Could you check a few things on this model? Use its own coordinates, in mm. Face numbers are marked on the shaded views. A direction names the side the tool comes from. Round coordinates to 2 decimals unless told otherwise and drop trailing zeros. Write each loop counter-clockwise with the first axis right and the second up, starting at its lowest first coordinate (ties: lowest second). Pieces come first, ordered by that corner, then holes. Notation, with made-up numbers: (-21.75, -19.75) - (28.25, -19.75) arc R5 ccw to (28.25, -15.75) - close; hole circle Ø5 at (16, 16). An arc over 180 degrees is marked (long way). Put each result on its own line as item: value.
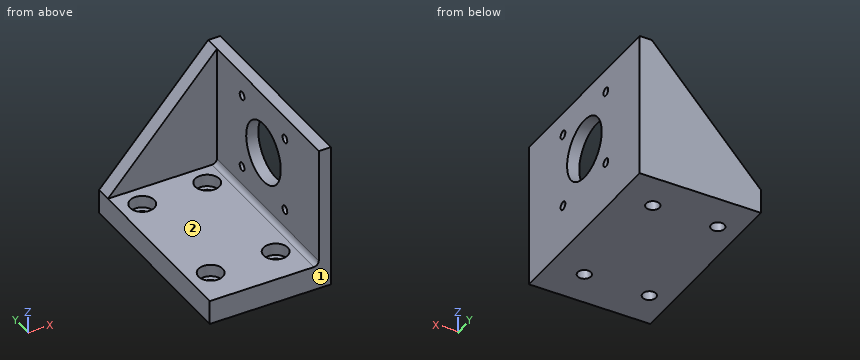
from build123d import *

# Parameters (mm, degrees)
SKETCH1_W                      = 50
SKETCH1_H                      = 80
BOSS_EXTRUDE1_DEPTH            = 10
SKETCH2_W                      = 5
SKETCH2_H                      = 80
BOSS_EXTRUDE2_DEPTH            = 50
SKETCH3_R                      = 12.5
CUT_EXTRUDE1_DEPTH             = 88.749643874
M3_CLEARANCE_HOLE1_D           = 3.4
CBORE_FOR_M5_SHCS1_D           = 5.5
CBORE_FOR_M5_SHCS1_CBORE_D     = 10
CBORE_FOR_M5_SHCS1_CBORE_DEPTH = 5
FILLET11_R                     = 2
BOSS_EXTRUDE3_DEPTH            = 6.35


with BuildPart() as part:
    # Sketch1 → Boss-Extrude1 (new body)
    with BuildSketch(Plane.XY):
        Rectangle(SKETCH1_W, SKETCH1_H)
    extrude(amount=BOSS_EXTRUDE1_DEPTH)

    # Sketch2 → Boss-Extrude2 (add)
    with BuildSketch(Plane.XY.offset(10)):
        with Locations((22.5, 0)):
            Rectangle(SKETCH2_W, SKETCH2_H)
    extrude(amount=BOSS_EXTRUDE2_DEPTH)

    # Sketch3 → Cut-Extrude1 (cut, through all)
    with BuildSketch(Plane(origin=(25, 0, 0), x_dir=(0, 0, -1), z_dir=(1, 0, 0))):
        with Locations((-35, 0)):
            Circle(SKETCH3_R)
    extrude(amount=-CUT_EXTRUDE1_DEPTH, mode=Mode.SUBTRACT)

    # M3 Clearance Hole1 (through all)
    with Locations(Plane(origin=(25, 0, 0), x_dir=(0, 0, -1), z_dir=(1, 0, 0))):
        with Locations((-50.5, -15.5), (-35, 0), (-50.5, 15.5), (-19.5, -15.5), (-19.5, 15.5)):
            Hole(M3_CLEARANCE_HOLE1_D / 2)

    # CBORE for M5 SHCS1 (through all)
    with Locations(Plane.XY.offset(10)):
        with Locations((-15.902931391, 24.76), (10.902931391, 24.76), (-15.902931391, -24.76), (10.902931391, -24.76)):
            CounterBoreHole(CBORE_FOR_M5_SHCS1_D / 2, CBORE_FOR_M5_SHCS1_CBORE_D / 2, CBORE_FOR_M5_SHCS1_CBORE_DEPTH)

    # Fillet11
    fillet11_edges = [part.edges().sort_by_distance(p)[0] for p in [
        (20, 0, 10),
    ]]
    fillet(fillet11_edges, radius=FILLET11_R)

    # Sketch8 → Boss-Extrude3 (add)
    with BuildSketch(Plane(origin=(0, 40, 0), x_dir=(1, 0, 0), z_dir=(0, 1, 0))):
        Polygon((-25, -10), (20, -60), (20, -10), align=None)
    extrude(amount=-BOSS_EXTRUDE3_DEPTH)


solid = part.part
(1) Please list where these lines run through material, in increasing order: probe 1 along Y at (x, z) = (23.6, 50.5); probe 2 along X at (y, z) = (24, 8); probe 3 along Z at (x, y) = (-13, 22.5). Write a range as from..to.
Values found:
probe 1: y = -40..-17.2, -13.8..13.8, 17.2..40
probe 2: x = -25..-20.84, -10.96..5.96, 15.84..25
probe 3: z = 0..5
(2) Imagine slicing it at B-B, the plane z = 35. List the corners of the cut face in (x, y) for me, then the cut area to 3 significant figures.
Values found:
outline: (-2.5, 33.65) - (20, 33.65) - (20, 12.5) - (25, 12.5) - (25, 40) - (-2.5, 40) - close; (20, -40) - (25, -40) - (25, -12.5) - (20, -12.5) - close
area: 418 mm^2
(3) Imagine slicing it at C-C, the plane y = 0. List the corners of the cut face in (x, z) for me, then the cut area to 3 significant figures.
Values found:
outline: (-25, 0) - (25, 0) - (25, 22.5) - (20, 22.5) - (20, 12) arc R2 cw to (18, 10) - (-25, 10) - close; (20, 47.5) - (25, 47.5) - (25, 60) - (20, 60) - close
area: 626 mm^2
(4) For the marked faces 1 and 2, which set-ups out of +Z, -Z, +X, -X, +Y, -Y let a thin tool reach every point of the face, with its end or its side?
Values found:
face 1: +Z, -Z, +X, -X, -Y
face 2: +Z, -X, -Y
(5) Imagine slicing it at D-D, the plane z = 19.5. List the corners of the cut face in (x, y) for me.
Values found:
outline: (-16.45, 33.65) - (20, 33.65) - (20, 17.2) - (25, 17.2) - (25, 40) - (-16.45, 40) - close; (20, -40) - (25, -40) - (25, -17.2) - (20, -17.2) - close; (20, -13.8) - (25, -13.8) - (25, 13.8) - (20, 13.8) - close
(6) Imagine slicing it at A-A, the plane y = -15.5. List the corners of the cut face in (x, z) for me, then the cut area to 3 significant figures.
Values found:
outline: (-25, 0) - (25, 0) - (25, 17.8) - (20, 17.8) - (20, 12) arc R2 cw to (18, 10) - (-25, 10) - close; (20, 21.2) - (25, 21.2) - (25, 48.8) - (20, 48.8) - close; (20, 52.2) - (25, 52.2) - (25, 60) - (20, 60) - close
area: 717 mm^2
(7) I'm going to push flat-ended pins straight in: pin 1 (5.5 mm diameter, centred on y = -15.5, z = 19.5, fed in from -X); pin 2 (5 mm diameter, centred on x = 10.9, y = 24.76, fed in from +Z); pin 3 (5 mm diameter, centred on x = -14.5, y = -23, fed in from +Z); pin 4 (8 mm diameter, centred on x = -5.5, y = -2, fed in from +Z). Where does each tip first touch, or does it pass through?
Values found:
pin 1: stops at x = 20
pin 2: passes through
pin 3: stops at z = 5
pin 4: stops at z = 10
